```python
from build123d import *

# Parameters (mm, degrees)
SKETCH1_R           = 1.002175573
BOSS_EXTRUDE1_DEPTH = 2


with BuildPart() as part:
    # Sketch1 → Boss-Extrude1 (new body)
    with BuildSketch(Plane.XY):
        with BuildLine():
            Line((-45.505390048, 11.932639401), (-2.959655608, 11.932639401))
            ThreePointArc((-2.959655608, 11.932639401), (-1.898995436, 12.371979229), (-1.459655608, 13.432639401))
            Line((-1.459655608, 13.432639401), (-1.459655608, 37.443224784))
            ThreePointArc((-1.459655608, 37.443224784), (-1.898995436, 38.503884956), (-2.959655608, 38.943224784))
            Line((-2.959655608, 38.943224784), (-45.505390048, 38.943224784))
            ThreePointArc((-45.505390048, 38.943224784), (-46.56605022, 38.503884956), (-47.005390048, 37.443224784))
            Line((-47.005390048, 37.443224784), (-47.005390048, 13.432639401))
            ThreePointArc((-47.005390048, 13.432639401), (-46.56605022, 12.371979229), (-45.505390048, 11.932639401))
        make_face()
        with Locations((-36.094331879, 34.905234601)):
            Circle(SKETCH1_R, mode=Mode.SUBTRACT)
        with Locations((-7.410237048, 14.298412667)):
            Circle(SKETCH1_R, mode=Mode.SUBTRACT)
    extrude(amount=-BOSS_EXTRUDE1_DEPTH)


solid = part.part
```
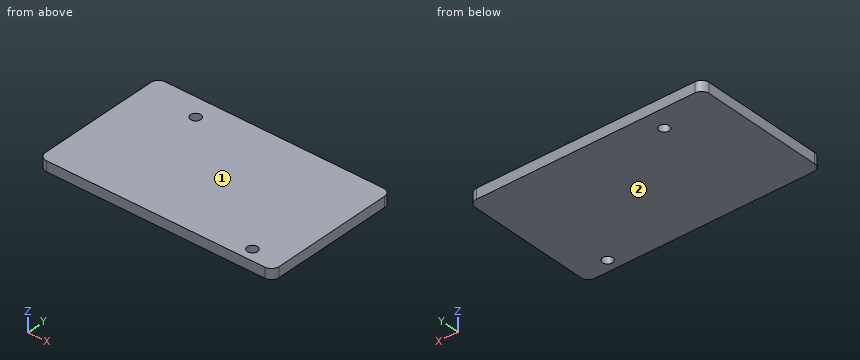
Source: CAD feature listing. Evaluate the final solid. Frame: model axes, mm. Face numbers are marked on the shaded views. Round coordinates to 2 decimals unless told otherwise and drop trailing zeros. Order: outer loops, then holes, each group sorted by start corner. A loop starts at its lowest first (then second) coordinate and runs counter-clockwise, first axis right, second up. Notation, with made-up numbers: (73.25, 52.5) -> (113.25, 52.5) arc R20 ccw to (113.25, 82.5) -> close; hole circle Ø5 at (77.25, 89.25). An arc over 180 degrees is marked (long way). Use CSV: the item, a comma, the result in double quotes.
(1) Pull-direction query (Z, two-part tool) for the marked faces 1 and 2; classes: +Z half, -Z half, draft (parallel to the pull), parting line (faces both ways), or undercut.
Report:
face 1,"+Z half"
face 2,"-Z half"
(2) Section A-A on x = -7. Return the cut outline in (y, z), and give its area (3 significant figures).
Report:
outline,"(11.93, -2) -> (13.38, -2) -> (13.38, 0) -> (11.93, 0) -> close; (15.21, -2) -> (38.94, -2) -> (38.94, 0) -> (15.21, 0) -> close"
area,"50.4 mm^2"
(3) Ray query, L1, parallel to Y at x = -37, z = -0.9. Return the intervals inside material, ascending.
Report:
L1,"11.93 to 34.48, 35.33 to 38.94"
